The listing builds one solid part. Answer for the finished solid, in the listing's coordinates (mm). A direction names the side the tool comes from. Coordinates: 2 decimals unless noted, no trailing zeros. Order: outer loops, then holes, each group sorted by start corner. A loop starts at its lowest first (then second) coordinate and runs counter-clockwise, first axis right, second up. Notation, with made-up numbers: (84.25, 26) -> (98.25, 26) arc R22 cw to (98.25, 54) -> close; hole circle Ø4 at (62, 75.5). An arc over 180 degrees is marked (long way). Return JSON: item names as keys, results as strings.
from build123d import *

# Parameters (mm, degrees)
EXTRUDE_1_DEPTH     = 17
CUT_EXTRUDE_START   = 30
SKETCH_2_W          = 12.8
SKETCH_2_H          = 24.4
CUT_EXTRUDE_1_DEPTH = 27.2
CUT_EXTRUDE_2_REACH = 47.706
SKETCH_3_R          = 2
CUT_EXTRUDE_3_REACH = 47.706
SKETCH_4_R          = 2


with BuildPart() as part:
    # 草图1 → 凸台-拉伸1 (new body)
    with BuildSketch(Plane(origin=(0, 0, 0), x_dir=(0, 0, -1), z_dir=(1, 0, 0))):
        Polygon((0, 0), (-30, 0), (-30, 2.8), (-27.2, 2.8), (-2.8, 27.2), (-2.8, 30), (0, 30), align=None)
    extrude(amount=EXTRUDE_1_DEPTH)

    # 草图2 → 切除-拉伸1 (cut)
    with BuildSketch(Plane(origin=(0, 0, 0), x_dir=(1, 0, 0), z_dir=(0, 1, 0)).offset(CUT_EXTRUDE_START)):
        with Locations((8.5, -15)):
            Rectangle(SKETCH_2_W, SKETCH_2_H)
    extrude(amount=-CUT_EXTRUDE_1_DEPTH, mode=Mode.SUBTRACT)

    # 草图3 → 切除-拉伸2 (cut, up to next)
    with BuildSketch(Plane(origin=(0, 0, 0), x_dir=(1, 0, 0), z_dir=(0, 1, 0)), mode=Mode.PRIVATE) as cut_extrude_2_sk1:
        with Locations(Location((8.5, -22, 0), (0, 0, 90))):
            Circle(SKETCH_3_R)
    cut_extrude_2_tool1 = extrude(cut_extrude_2_sk1.sketch, amount=CUT_EXTRUDE_2_REACH, mode=Mode.PRIVATE) & part.part
    # 草图3 → 切除-拉伸2 (cut, up to next)
    with BuildSketch(Plane(origin=(0, 0, 0), x_dir=(1, 0, 0), z_dir=(0, 1, 0)), mode=Mode.PRIVATE) as cut_extrude_2_sk2:
        with Locations(Location((8.5, -13, 0), (0, 0, 90))):
            Circle(SKETCH_3_R)
    cut_extrude_2_tool2 = extrude(cut_extrude_2_sk2.sketch, amount=CUT_EXTRUDE_2_REACH, mode=Mode.PRIVATE) & part.part
    add(cut_extrude_2_tool1.solids().sort_by_distance((8.5, 0, 22))[0], mode=Mode.SUBTRACT)
    add(cut_extrude_2_tool2.solids().sort_by_distance((8.5, 0, 13))[0], mode=Mode.SUBTRACT)

    # 草图4 → 切除-拉伸3 (cut, up to next)
    with BuildSketch(Plane.XY, mode=Mode.PRIVATE) as cut_extrude_3_sk1:
        with Locations(Location((8.5, 22, 0), (0, 0, 90))):
            Circle(SKETCH_4_R)
    cut_extrude_3_tool1 = extrude(cut_extrude_3_sk1.sketch, amount=CUT_EXTRUDE_3_REACH, mode=Mode.PRIVATE) & part.part
    # 草图4 → 切除-拉伸3 (cut, up to next)
    with BuildSketch(Plane.XY, mode=Mode.PRIVATE) as cut_extrude_3_sk2:
        with Locations(Location((8.5, 13, 0), (0, 0, 90))):
            Circle(SKETCH_4_R)
    cut_extrude_3_tool2 = extrude(cut_extrude_3_sk2.sketch, amount=CUT_EXTRUDE_3_REACH, mode=Mode.PRIVATE) & part.part
    add(cut_extrude_3_tool1.solids().sort_by_distance((8.5, 22, 0))[0], mode=Mode.SUBTRACT)
    add(cut_extrude_3_tool2.solids().sort_by_distance((8.5, 13, 0))[0], mode=Mode.SUBTRACT)


solid = part.part
1. Determine the mould class of faces 1 (the face through (7.148, 20.526, 1.38)), 2 (the face through (17, 9, 8)), 3 (the face through (1, 15, 15)) for opening direction X: pulls with the +X half, pulls with the -X half, needs draft (parallel to the pull), parting line crosses it, or undercut.
Answer block:
{"face 1": "undercut", "face 2": "pulls with the +X half", "face 3": "needs draft"}
2. The part is cut by section C-C on x = 8.5. Give the vertices of the cut face in (y, z).
Answer block:
{"outline": "(0, 0) -> (11, 0) -> (11, 2.8) -> (2.8, 2.8) -> (2.8, 11) -> (0, 11) -> close; (0, 15) -> (2.8, 15) -> (2.8, 20) -> (0, 20) -> close; (0, 24) -> (2.8, 24) -> (2.8, 30) -> (0, 30) -> close; (15, 0) -> (20, 0) -> (20, 2.8) -> (15, 2.8) -> close; (24, 0) -> (30, 0) -> (30, 2.8) -> (24, 2.8) -> close"}
3. Consider line 1 (Y direction, x = 8.5, z = 2); line 2 (X direction, y = 2.05, z = 22). Determine where each line is inside the solid, lowest interval first. Write a range as from..to.
Answer block:
{"line 1": "y = 0..11, 15..20, 24..30", "line 2": "x = 0..6.5, 10.5..17"}
4. The part is cut by section A-A on z = 13. Give the vertices of the cut face in (x, y), and give its area (3 significant figures).
Answer block:
{"outline": "(0, 0) -> (6.5, 0) -> (6.5, 2.8) -> (2.1, 2.8) -> (2.1, 17) -> (0, 17) -> close; (10.5, 0) -> (17, 0) -> (17, 17) -> (14.9, 17) -> (14.9, 2.8) -> (10.5, 2.8) -> close", "area": "96.0 mm2"}
5. For faces 4 (the face through (7.148, 1.38, 14.474)), 5 (the face through (8, 16, 2.8)), determine the directions among +Z, -Z, +X, -X, +Y, -Y from which every point of the face is accessible in a straight line to the end or side of a thin tool.
Answer block:
{"face 4": "+Y, -Y", "face 5": "+Z, +Y"}
6. The part is cut by section D-D on z = 19. Give the vertices of the cut face in (x, y).
Answer block:
{"outline": "(0, 0) -> (17, 0) -> (17, 11) -> (14.9, 11) -> (14.9, 2.8) -> (2.1, 2.8) -> (2.1, 11) -> (0, 11) -> close"}
7. Each of these flat-tipped pins is pushed along its axis until it touches: pin 1 Ø3.5 at (x, z) = (8.5, 22) entering from -Y; pin 2 Ø8.5 at (x, z) = (10.5, 17) entering from +Y. Where does it stop, or does it pass through?
Answer block:
{"pin 1": "passes through", "pin 2": "stops at y = 2.8"}
